from build123d import *

# Parameters (mm, degrees)
F0_W     = 190.5
F0_H     = 127
F1_DEPTH = 127
F2_W     = 381
F2_H     = 889
F3_DEPTH = 127
F4_W     = 127
F4_H     = 635
F5_DEPTH = 381
F7_DEPTH = 381.001


with BuildPart() as f1:
    # F0 (on Top) → F1 (new body)
    with BuildSketch(Plane.XY):
        Polygon((79.417029, 127), (79.417029, 0), (714.417029, 0), (714.417029, 508), (79.417029, 508), align=None)
        with Locations((-15.832971, 63.5)):
            Rectangle(F0_W, F0_H)
    extrude(amount=F1_DEPTH)

    # F2 (on face) → F3 (join)
    with BuildSketch(Plane(origin=(0, 508, 0), x_dir=(-1, 0, 0), z_dir=(0, 1, 0))):
        with Locations((-523.917029, 571.5)):
            Rectangle(F2_W, F2_H)
        Polygon((-333.417029, 1016), (-333.417029, 127), (-79.417029, 127), align=None)
    extrude(amount=-F3_DEPTH)

    # F4 (on face) → F5 (join, through all)
    with BuildSketch(Plane.XZ.offset(-381)):
        with Locations((396.917029, 444.5)):
            Rectangle(F4_W, F4_H)
    extrude(amount=F5_DEPTH)

    # F6 (on face) → F7 (cut, through all)
    with BuildSketch(Plane(origin=(333.417029, 0, 0), x_dir=(0, -1, 0), z_dir=(-1, 0, 0))):
        Polygon((0, 762), (-381, 762), (0, 127), align=None)
    extrude(amount=-F7_DEPTH, mode=Mode.SUBTRACT)


solid = f1.part
Verification items for the finished model (mm, model axes). A direction names the side the tool comes from. Round coordinates to 2 decimals unless told otherwise and drop trailing zeros. Order: outer loops, then holes, each group sorted by start corner. A loop starts at its lowest first (then second) coordinate and runs counter-clockwise, first axis right, second up.
1. Go/stop test with flat-tipped pins: P1, Ø8, axis at x = 484.5, z = 711, coming from the -Y side; P2, Ø2, axis at x = 396.5, z = 632.5, coming from the -Y side; P3, Ø2, axis at y = 365.5, z = 451, coming from the +X side. Record where each tip stops, or that it passes through.
Final values:
P1: stops at y = 381
P2: stops at y = 302.7
P3: stops at x = 460.42
2. Section check B-B on x = 432.5. Record the cut outline in (y, z).
Final values:
outline: (0, 0) - (508, 0) - (508, 1016) - (381, 1016) - (381, 762) - (0, 127) - close
3. Thickness scan on L1, parallel to X at y = 340.5, z = 318; L2, parallel to Z at x = 611, y = 98.5; L3, parallel to Y at x = 671, z = 343.5. Record the ranges inside material, lowest first.
Final values:
L1: x = 333.42 to 460.42
L2: z = 0 to 127
L3: y = 381 to 508
4. Section check D-D on x = 278.5. Record the cut outline in (y, z), then the cut area to 3 significant figures.
Final values:
outline: (0, 0) - (508, 0) - (508, 823.79) - (381, 823.79) - (381, 127) - (0, 127) - close
area: 153,000 mm2
5. Access from +Z, -Z, +X, -X, +Y, -Y to the whole of each face (thin tool, end or side, straight path). Record for faces 1 (the flat face through (472, 381, 578)), 2 (the flat face through (157, 151, 127)), 3 (the flat face through (79.417, 320, 63)), 4 (the flat face through (460.417, 236, 369)).
Final values:
face 1: +Z, -Y
face 2: +Z, -X, -Y
face 3: +Z, -Z, -X, +Y
face 4: +Z, +X, -Y
6. Section check A-A on y = 270. Record the cut outline in (x, z).
Final values:
outline: (79.42, 0) - (714.42, 0) - (714.42, 127) - (460.42, 127) - (460.42, 577) - (333.42, 577) - (333.42, 127) - (79.42, 127) - close
7. Section check C-C on z = 288. Record the cut outline in (x, y).
Final values:
outline: (125.42, 381) - (333.42, 381) - (333.42, 96.6) - (460.42, 96.6) - (460.42, 381) - (714.42, 381) - (714.42, 508) - (125.42, 508) - close
